Model file for the job. Use its own axes, mm. Round coordinates to 2 decimals unless told otherwise and drop trailing zeros. Loops run counter-clockwise (first coordinate to the right, second up) from the corner with the lowest first, then second, coordinate; pieces in that order, holes last. Notation, with made-up numbers: (21, 7) -> (40, 7) arc R29 cw to (40, 27) -> close; hole circle Ø4 at (66.5, 28). An arc over 180 degrees is marked (long way). Use a Markdown table: item, result. Add a question column.
```python
from build123d import *

# Parameters (mm, degrees)
SKETCH1_R            = 64.4
BOSS_EXTRUDE1_DEPTH  = 1.5
M6_CLEARANCE_HOLE1_D = 6.6
CIRPATTERN2_COUNT    = 4
M4_CLEARANCE_HOLE1_D = 4.3
CIRPATTERN1_COUNT    = 4
SKETCH10_R           = 43.25
CUT_EXTRUDE1_DEPTH   = 92.124749657


with BuildPart() as part:
    # Sketch1 → Boss-Extrude1 (new, symmetric)
    with BuildSketch(Plane(origin=(0, 0, 0), x_dir=(1, 0, 0), z_dir=(0, 1, 0))):
        with Locations(Location((0, 0, 0), (0, 0, 270))):
            Circle(SKETCH1_R)
    extrude(amount=BOSS_EXTRUDE1_DEPTH, both=True)

    # M6 Clearance Hole1 (through all)
    with Locations(Plane(origin=(0, 1.5, 0), x_dir=(1, 0, 0), z_dir=(0, 1, 0))):
        with Locations((54.4, 0)):
            m6_clearance_hole1 = Hole(M6_CLEARANCE_HOLE1_D / 2)

    # CirPattern2: M6 Clearance Hole1 ×4 about axis
    cirpattern2_axis = Axis((0, 0, 0), (0, 1, 0))
    for i in range(1, CIRPATTERN2_COUNT):
        add(m6_clearance_hole1.rotate(cirpattern2_axis, i * 360 / CIRPATTERN2_COUNT), mode=Mode.SUBTRACT)

    # M4 Clearance Hole1 (through all)
    with Locations(Plane(origin=(0, 1.5, 0), x_dir=(1, 0, 0), z_dir=(0, 1, 0))):
        with Locations((38.466608897, 38.466608897)):
            m4_clearance_hole1 = Hole(M4_CLEARANCE_HOLE1_D / 2)

    # CirPattern1: M4 Clearance Hole1 ×4 about axis
    cirpattern1_axis = Axis((0, 0, 0), (0, 1, 0))
    for i in range(1, CIRPATTERN1_COUNT):
        add(m4_clearance_hole1.rotate(cirpattern1_axis, i * 360 / CIRPATTERN1_COUNT), mode=Mode.SUBTRACT)

    # Sketch10 → Cut-Extrude1 (cut, through all)
    with BuildSketch(Plane(origin=(0, 1.5, 0), x_dir=(1, 0, 0), z_dir=(0, 1, 0))):
        with Locations(Location((0, 0, 0), (0, 0, 270))):
            Circle(SKETCH10_R)
    extrude(amount=-CUT_EXTRUDE1_DEPTH, mode=Mode.SUBTRACT)


solid = part.part
```
1) Pin check, flat tips, straight feed: pin 1 Ø1.5 at (x, y) = (29.5, 1) entering from +Z; pin 2 Ø1 at (y, z) = (1, -11.5) entering from -X; pin 3 Ø1 at (x, y) = (-4, 0.5) entering from -Z. Stop position of each tip, or through.
2) Cut at C-C on z = 30. Write the cut outline in (x, y), and give its area (3 significant figures).
3) Cut at A-A on z = 0. Write the cut outline in (x, y), and give its area (3 significant figures).
4) Wall check: probe 1 along X at (y, z) = (-1.1, 2); probe 2 along Z at (x, y) = (-3, 1.3); probe 3 along X at (y, z) = (-1.15, 38.5). Give the ranges that are in metal, low to high. Write a range as from..to.
5) Pull direction Z, two halves, no side cores. Call faces 1 (the face through (0.1, 0, 57.7)), 2 (the face through (44, -1.5, -1)), 3 (the face through (-24.666, 0.021, 59.489)): +Z half, -Z half, draft (parallel to the pull), parting line (faces both ways), or undercut.
6) Cut at D-D on x = -54.4. Write the cut outline in (y, z), and give its area (3 significant figures).
7) Cut at B-B on x = 0. Write the cut outline in (y, z).
Established:
| question | item | result |
|---|---|---|
| 1 | pin 1 | stops at z = 57.63 |
| 1 | pin 2 | stops at x = -63.45 |
| 1 | pin 3 | stops at z = -64.3 |
| 2 | outline | (-56.99, -1.5) -> (-31.15, -1.5) -> (-31.15, 1.5) -> (-56.99, 1.5) -> close; (31.15, -1.5) -> (56.99, -1.5) -> (56.99, 1.5) -> (31.15, 1.5) -> close |
| 2 | area | 155 mm^2 |
| 3 | outline | (-64.4, -1.5) -> (-57.7, -1.5) -> (-57.7, 1.5) -> (-64.4, 1.5) -> close; (-51.1, -1.5) -> (-43.25, -1.5) -> (-43.25, 1.5) -> (-51.1, 1.5) -> close; (43.25, -1.5) -> (51.1, -1.5) -> (51.1, 1.5) -> (43.25, 1.5) -> close; (57.7, -1.5) -> (64.4, -1.5) -> (64.4, 1.5) -> (57.7, 1.5) -> close |
| 3 | area | 87.3 mm^2 |
| 4 | probe 1 | x = -64.37..-57.02, -51.78..-43.2, 43.2..51.78, 57.02..64.37 |
| 4 | probe 2 | z = -64.33..-55.77, -53.03..-43.15, 43.15..53.03, 55.77..64.33 |
| 4 | probe 3 | x = -51.62..-40.62, -36.32..-19.71, 19.71..36.32, 40.62..51.62 |
| 5 | face 1 | undercut |
| 5 | face 2 | draft |
| 5 | face 3 | parting line |
| 6 | outline | (-1.5, -34.47) -> (1.5, -34.47) -> (1.5, -3.3) -> (-1.5, -3.3) -> close; (-1.5, 3.3) -> (1.5, 3.3) -> (1.5, 34.47) -> (-1.5, 34.47) -> close |
| 6 | area | 187 mm^2 |
| 7 | outline | (-1.5, -64.4) -> (1.5, -64.4) -> (1.5, -57.7) -> (-1.5, -57.7) -> close; (-1.5, -51.1) -> (1.5, -51.1) -> (1.5, -43.25) -> (-1.5, -43.25) -> close; (-1.5, 43.25) -> (1.5, 43.25) -> (1.5, 51.1) -> (-1.5, 51.1) -> close; (-1.5, 57.7) -> (1.5, 57.7) -> (1.5, 64.4) -> (-1.5, 64.4) -> close |
